Check sheet for the modelled part. Datum: model origin and axes. Units: mm. A direction names the side the tool comes from. Coordinates: 2 decimals unless noted, no trailing zeros. Write each loop counter-clockwise with the first axis right and the second up, starting at its lowest first coordinate (ties: lowest second). Pieces come first, ordered by that corner, then holes. Notation, with made-up numbers: (61, 36.25) - (106, 36.25) arc R26 ccw to (106, 55.25) - close; hole circle Ø9 at (-16, -15.5). An arc over 180 degrees is marked (long way). Use one line per item in the form item = value. Start each with the question number.
1. Go/stop test with a flat-tipped pin: pin 1 Ø2 at (x, z) = (15, 0.5) entering from -Y. Record where the tip stops, or that it passes through.
2. Draft check along Z on faces 3 (the face through (0, 2, 0)), 4 (the face through (22.5, 3, 0)), 5 (the face through (0, 3, 4.75)), 6 (the face through (0, 3, -4.75)). Enter one of: +Z half, -Z half, draft (parallel to the pull), parting line (faces both ways), or undercut.
3. Cross-section at A-A on z = 0. Record the boundary of the cut face in (x, y).
4. Cross-section at C-C on y = 1. Record the boundary of the cut face in (x, z), then the cut area to 3 significant figures.
5. Cross-section at D-D on y = 3.5. Record the boundary of the cut face in (x, z), then the cut area to 3 significant figures.
6. Tool access check on faces 1 (the face through (-22.5, 3, 0)), 2 (the face through (0, 4, -1)). Record the directions out of +Z, -Z, +X, -X, +Y, -Y that give a thin tool (end or side, any length) a straight path to the whole face; none if there is none.
7. Scan lines: line 1 along Z through (x, y) = (20.5, 3); line 2 along Z through (x, y) = (13.5, 5.75); line 3 along Y through (x, z) = (-5.5, 1.25). Record each from-to range of solid material in increasing order.
8. Cross-section at B-B on x = -20.5. Record the boundary of the cut face in (y, z), then the cut area to 4 significant figures.
```python
from build123d import *

# Parameters (mm, degrees)
SKETCH1_W            = 45
SKETCH1_H            = 9.5
SKETCH1_W_2          = 36.6
SKETCH1_H_2          = 2
BOSS_EXTRUDE1_DEPTH  = 6.5
SKETCH2_W            = 45
SKETCH2_H            = 9.5
BOSS_EXTRUDE2_DEPTH  = 2
M2_CLEARANCE_HOLE1_D = 2.4
SKETCH5_R            = 0.4
BOSS_EXTRUDE3_DEPTH  = 3.5


with BuildPart() as part:
    # Sketch1 → Boss-Extrude1 (new body)
    with BuildSketch(Plane(origin=(0, 0, 0), x_dir=(1, 0, 0), z_dir=(0, 1, 0))):
        Rectangle(SKETCH1_W, SKETCH1_H)
        Rectangle(SKETCH1_W_2, SKETCH1_H_2, mode=Mode.SUBTRACT)
    extrude(amount=BOSS_EXTRUDE1_DEPTH)

    # Sketch2 → Boss-Extrude2 (add)
    with BuildSketch(Plane.XZ):
        Rectangle(SKETCH2_W, SKETCH2_H)
    extrude(amount=-BOSS_EXTRUDE2_DEPTH)

    # M2 Clearance Hole1 (through all)
    with Locations(Plane(origin=(0, 6.5, 0), x_dir=(1, 0, 0), z_dir=(0, 1, 0))):
        with Locations((20.5, 0), (-20.5, 0)):
            Hole(M2_CLEARANCE_HOLE1_D / 2)

    # Sketch5 → Boss-Extrude3 (add)
    with BuildSketch(Plane.XZ):
        with Locations(Location((-21.75, 2, 0), (0, 0, 270))):
            Circle(SKETCH5_R)
        with Locations(Location((-21.75, -2, 0), (0, 0, 270))):
            Circle(SKETCH5_R)
        with Locations(Location((21.75, -2, 0), (0, 0, 270))):
            Circle(SKETCH5_R)
    extrude(amount=BOSS_EXTRUDE3_DEPTH)


solid = part.part
```
Final values:
q1.pin_1 = 0
q2.face_3 = undercut
q2.face_4 = draft
q2.face_5 = +Z half
q2.face_6 = -Z half
q3.outline = (-22.5, 0) - (-21.7, 0) - (-21.7, 6.5) - (-22.5, 6.5) - close; (-19.3, 0) - (19.3, 0) - (19.3, 6.5) - (18.3, 6.5) - (18.3, 2) - (-18.3, 2) - (-18.3, 6.5) - (-19.3, 6.5) - close; (21.7, 0) - (22.5, 0) - (22.5, 6.5) - (21.7, 6.5) - close
q4.outline = (-22.5, -4.75) - (22.5, -4.75) - (22.5, 4.75) - (-22.5, 4.75) - close; hole circle Ø2.4 at (-20.5, 0); hole circle Ø2.4 at (20.5, 0)
q4.area = 418 mm²
q5.outline = (-22.5, -4.75) - (22.5, -4.75) - (22.5, 4.75) - (-22.5, 4.75) - close; hole circle Ø2.4 at (-20.5, 0); hole (-18.3, -1) - (18.3, -1) - (18.3, 1) - (-18.3, 1) - close; hole circle Ø2.4 at (20.5, 0)
q5.area = 345 mm²
q6.face_1 = +Z, -Z, -X, +Y, -Y
q6.face_2 = +Y
q7.line_1 = -4.75 to -1.2, 1.2 to 4.75
q7.line_2 = -4.75 to -1, 1 to 4.75
q7.line_3 = 0 to 6.5
q8.outline = (0, -4.75) - (6.5, -4.75) - (6.5, -1.2) - (0, -1.2) - close; (0, 1.2) - (6.5, 1.2) - (6.5, 4.75) - (0, 4.75) - close
q8.area = 46.15 mm²
